Geometry check sheet. Reference: the model listing, model coordinates, mm. Face numbers are marked on the shaded views. A direction names the side the tool comes from. Coordinates: 2 decimals unless noted, no trailing zeros. Order: outer loops, then holes, each group sorted by start corner. A loop starts at its lowest first (then second) coordinate and runs counter-clockwise, first axis right, second up. Notation, with made-up numbers: (37.25, 65.25) - (43.25, 65.25) arc R16 ccw to (43.25, 80.25) - close; hole circle Ø8 at (79, 72). An arc over 180 degrees is marked (long way). Return JSON: item names as keys, results as strings. Group by question number.
Item 1: Tool access check on the marked faces 1, 2, 3 and 4. Record the directions out of +Z, -Z, +X, -X, +Y, -Y that give a thin tool (end or side, any length) a straight path to the whole face; none if there is none.
Item 2: Section check A-A on x = 0. Enter the section's corners in (y, z), then the cut area to 3 significant figures.
Item 3: Scan lines: probe 1 along X at (y, z) = (2.45, 0); probe 2 along X at (y, z) = (-25, 7.5); probe 3 along Z at (x, y) = (-20, 1.7). Record each from-to range of solid material in increasing order.
Item 4: Section check D-D on y = 1. Enter the section's corners in (x, z).
Item 5: Section check C-C on z = -5. Enter the section's corners in (x, y), then the cut area to 3 significant figures.
Item 6: Section check B-B on y = -25. Enter the section's corners in (x, z), then the cut area to 3 significant figures.
Item 7: Gauge pin test, flat ends, axial feed: pin 1 (4 mm diameter, centred on y = -8.5, z = -11, fed in from +X); pin 2 (7 mm diameter, centred on x = -20, z = 0, fed in from +Y); pin 3 (8 mm diameter, centred on x = 18, z = 3, fed in from -Y); pin 4 (2 mm diameter, centred on y = -23, z = 11, fed in from +X). Record the tip position at first contact, or that the pin passes through.
Item 8: Draft check along X on the marked faces 5, 6 and 7. Enter one of: pulls with the +X half, pulls with the -X half, needs draft (parallel to the pull), parting line crosses it, or undercut.
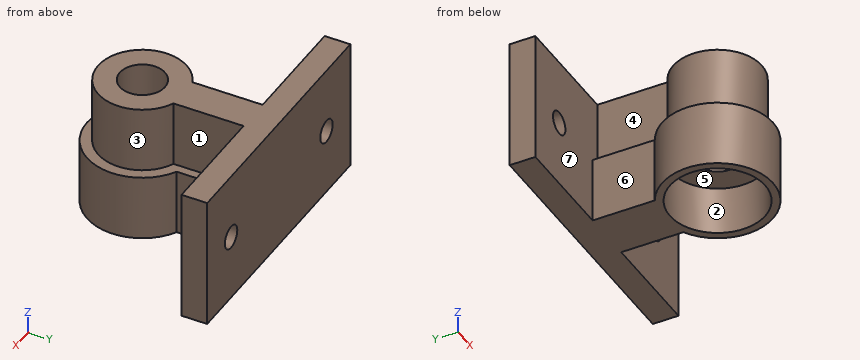
from build123d import *

# Parameters (mm, degrees)
SKETCH1_W           = 60
SKETCH1_H           = 30
BOSS_EXTRUDE1_DEPTH = 5.8
SKETCH2_R           = 2.6
CUT_EXTRUDE1_DEPTH  = 6
SKETCH3_R           = 5.1
BOSS_EXTRUDE2_DEPTH = 15
BOSS_EXTRUDE3_START = -15
SKETCH4_R           = 5.1
BOSS_EXTRUDE3_DEPTH = 15
SKETCH5_R           = 10.75
CUT_EXTRUDE2_DEPTH  = 11


with BuildPart() as part:
    # Sketch1 → Boss-Extrude1 (new body)
    with BuildSketch(Plane(origin=(0, 0, 0), x_dir=(1, 0, 0), z_dir=(0, 1, 0))):
        Rectangle(SKETCH1_W, SKETCH1_H)
    extrude(amount=BOSS_EXTRUDE1_DEPTH)

    # Sketch2 → Cut-Extrude1 (cut)
    with BuildSketch(Plane(origin=(0, 0, 0), x_dir=(1, 0, 0), z_dir=(0, 1, 0))):
        with Locations(Location((-20, 0, 0), (0, 0, 270))):
            Circle(SKETCH2_R)
    cut_extrude1 = extrude(amount=CUT_EXTRUDE1_DEPTH, mode=Mode.SUBTRACT)

    # Mirror1: Cut-Extrude1 across plane
    add(cut_extrude1.mirror(Plane(origin=(0, 0, 0), x_dir=(0, 0, 1), z_dir=(1, 0, 0))), mode=Mode.SUBTRACT)

    # Sketch3 → Boss-Extrude2 (add)
    with BuildSketch(Plane.XY):
        with BuildLine():
            Line((-4, 0), (4, 0))
            Line((4, 0), (4, -15.83484861))
            ThreePointArc((4, -15.83484861), (0, -35), (-4, -15.83484861))
            Line((-4, -15.83484861), (-4, 0))
        make_face()
        with Locations((0, -25)):
            Circle(SKETCH3_R, mode=Mode.SUBTRACT)
    extrude(amount=BOSS_EXTRUDE2_DEPTH)

    # Sketch4 → Boss-Extrude3 (add)
    with BuildSketch(Plane.XY.offset(BOSS_EXTRUDE3_START)):
        with BuildLine():
            Line((-6, -14.0341439), (-6, 0))
            Line((-6, 0), (6, 0))
            Line((6, 0), (6, -14.0341439))
            ThreePointArc((6, -14.0341439), (0, -37.5), (-6, -14.0341439))
        make_face()
        with Locations((0, -25)):
            Circle(SKETCH4_R, mode=Mode.SUBTRACT)
    extrude(amount=BOSS_EXTRUDE3_DEPTH)

    # Sketch5 → Cut-Extrude2 (cut)
    with BuildSketch(Plane(origin=(0, 0, -15), x_dir=(-1, 0, 0), z_dir=(0, 0, -1))):
        with Locations((0, -25)):
            Circle(SKETCH5_R)
    extrude(amount=-CUT_EXTRUDE2_DEPTH, mode=Mode.SUBTRACT)


solid = part.part
Computed:
{
 "1": {"face 1": "+Z, +X", "face 2": "-Z", "face 3": "+Z", "face 4": "+Z, -X"},
 "2": {"outline": "(-37.5, -15) - (-35.75, -15) - (-35.75, -4) - (-30.1, -4) - (-30.1, 15) - (-35, 15) - (-35, 0) - (-37.5, 0) - close; (-19.9, -4) - (-14.25, -4) - (-14.25, -15) - (5.8, -15) - (5.8, 15) - (-19.9, 15) - close", "area": "831 mm²"},
 "3": {"probe 1": "x = -30 to -22.6, -17.4 to 17.4, 22.6 to 30", "probe 2": "x = -10 to -5.1, 5.1 to 10", "probe 3": "z = -15 to -2.6, 2.6 to 15"},
 "4": {"outline": "(-30, -15) - (30, -15) - (30, 15) - (-30, 15) - close; hole circle Ø5.2 at (-20, 0); hole circle Ø5.2 at (20, 0)"},
 "5": {"outline": "(-30, 0) - (-6, 0) - (-6, -14.03) arc R12.5 ccw (long way) to (6, -14.03) - (6, 0) - (30, 0) - (30, 5.8) - (-30, 5.8) - close; hole circle Ø21.5 at (0, -25)", "area": "632 mm²"},
 "6": {"outline": "(-12.5, -15) - (-10.75, -15) - (-10.75, -4) - (-5.1, -4) - (-5.1, 15) - (-10, 15) - (-10, 0) - (-12.5, 0) - close; (5.1, -4) - (10.75, -4) - (10.75, -15) - (12.5, -15) - (12.5, 0) - (10, 0) - (10, 15) - (5.1, 15) - close", "area": "245 mm²"},
 "7": {"pin 1": "stops at x = 6", "pin 2": "stops at y = 5.8", "pin 3": "stops at y = 0", "pin 4": "stops at x = 9.95"},
 "8": {"face 5": "undercut", "face 6": "pulls with the -X half", "face 7": "needs draft"}
}
